from build123d import *

# Parameters (mm, degrees)
F1_DEPTH = 10
F3_D     = 10
F4_R     = 18
F5_DEPTH = 30
F7_D     = 14
F7_DEPTH = 18
F7_TIP   = 4.2060243332


with BuildPart() as f1:
    # F0 (on Top) → F1 (new body, symmetric)
    with BuildSketch(Plane.XY):
        with BuildLine():
            ThreePointArc((10.7142857143, 22.5876975726), (21.1288563682, 13.3630620956), (25, 0))
            ThreePointArc((25, 0), (29.6547751618, 8.4515425473), (39.2857142857, 9.0350790291))
            Line((39.2857142857, 9.0350790291), (10.7142857143, 22.5876975726))
        make_face()
        with BuildLine():
            ThreePointArc((39.2857142857, -9.0350790291), (29.6547751618, -8.4515425473), (25, 0))
            ThreePointArc((25, 0), (21.1288563682, -13.3630620956), (10.7142857143, -22.5876975726))
            Line((10.7142857143, -22.5876975726), (39.2857142857, -9.0350790291))
        make_face()
        with BuildLine():
            ThreePointArc((-25, 0), (-21.1288563682, 13.3630620956), (-10.7142857143, 22.5876975726))
            Line((-10.7142857143, 22.5876975726), (-39.2857142857, 9.0350790291))
            ThreePointArc((-39.2857142857, 9.0350790291), (-29.6547751618, 8.4515425473), (-25, 0))
        make_face()
        with BuildLine():
            ThreePointArc((-39.2857142857, -9.0350790291), (-29.6547751618, -8.4515425473), (-25, 0))
            ThreePointArc((-25, 0), (-29.6547751618, 8.4515425473), (-39.2857142857, 9.0350790291))
            ThreePointArc((-39.2857142857, 9.0350790291), (-45, 0), (-39.2857142857, -9.0350790291))
        make_face()
        with BuildLine():
            ThreePointArc((39.2857142857, 9.0350790291), (29.6547751618, 8.4515425473), (25, 0))
            ThreePointArc((25, 0), (29.6547751618, -8.4515425473), (39.2857142857, -9.0350790291))
            ThreePointArc((39.2857142857, -9.0350790291), (43.4515425473, -5.3452248382), (45, 0))
            ThreePointArc((45, 0), (43.4515425473, 5.3452248382), (39.2857142857, 9.0350790291))
        make_face()
        with BuildLine():
            Line((-39.2857142857, -9.0350790291), (-10.7142857143, -22.5876975726))
            ThreePointArc((-10.7142857143, -22.5876975726), (-21.1288563682, -13.3630620956), (-25, 0))
            ThreePointArc((-25, 0), (-29.6547751618, -8.4515425473), (-39.2857142857, -9.0350790291))
        make_face()
        with BuildLine():
            ThreePointArc((10.7142857143, -22.5876975726), (21.1288563682, -13.3630620956), (25, 0))
            ThreePointArc((25, 0), (21.1288563682, 13.3630620956), (10.7142857143, 22.5876975726))
            ThreePointArc((10.7142857143, 22.5876975726), (0, 25), (-10.7142857143, 22.5876975726))
            ThreePointArc((-10.7142857143, 22.5876975726), (-21.1288563682, 13.3630620956), (-25, 0))
            ThreePointArc((-25, 0), (-21.1288563682, -13.3630620956), (-10.7142857143, -22.5876975726))
            ThreePointArc((-10.7142857143, -22.5876975726), (0, -25), (10.7142857143, -22.5876975726))
        make_face()
    extrude(amount=F1_DEPTH, both=True)

    # F3 (through all)
    with Locations(Plane.XY.offset(10)):
        with Locations((-35, 0), (35, 0)):
            Hole(F3_D / 2)

    # F4 (on face) → F5 (join)
    with BuildSketch(Plane.XY.offset(10)):
        Circle(F4_R)
    extrude(amount=F5_DEPTH)

    # F7
    with Locations(Plane.XY.offset(40)):
        with Locations((0, 0)):
            Hole(F7_D / 2, depth=F7_DEPTH)
            with Locations((0, 0, -(F7_DEPTH + F7_TIP / 2))):  # 118° drill point
                Cone(0, F7_D / 2, F7_TIP, mode=Mode.SUBTRACT)


solid = f1.part
Work out the finished part from the listing and answer in its coordinate system (mm). A direction names the side the tool comes from. Give positions to 0.01 mm unless a question says otherwise; leave off trailing zeros. Loops run counter-clockwise (first coordinate to the right, second up) from the corner with the lowest first, then second, coordinate; pieces in that order, holes last. Notation, with made-up numbers: (41, 38.25) - (61, 38.25) arc R21 cw to (61, 52.25) - close; hole circle Ø9 at (1.5, 84.25). An arc over 180 degrees is marked (long way). Answer in a Markdown table with one row per item.
(1) Section C-C (y = -4) is taken. State how many separate pieces and enclosed holes the cut face has, and give its area (3 significant figures).
Results list:
| item | result |
|---|---|
| separate pieces | 3 |
| enclosed holes | 0 |
| area | 2,360 mm² |
(2) Consider L1, parallel to Y at x = 0, z = 30; L2, parallel to Z at x = -28, y = 1; L3, parallel to Y at x = -35, z = -4. Determine where each line is inside the solid, lowest interval first. Write a range as [from, to].
Results list:
| item | result |
|---|---|
| L1 | y = [-18, -7], [7, 18] |
| L2 | z = [-10, 10] |
| L3 | y = [-11.07, -5], [5, 11.07] |
(3) For a pull along Y with two mould halves and no side action, classify faces 3 (the face through (-6.466, -2.681, 30.874)), 4 (the face through (-1, 0, -10)), 5 (the face through (-24.8, 15.906, 0.14)), 6 (the face through (0, -25, 0)) as pulls with the +Y half, pulls with the -Y half, needs draft (parallel to the pull), parting line crosses it, or undercut.
Results list:
| item | result |
|---|---|
| face 3 | undercut |
| face 4 | needs draft |
| face 5 | pulls with the +Y half |
| face 6 | pulls with the -Y half |
(4) A tool of negligible diameter and unlimited length cuts with its end or side. For faces 1 (the face through (-2.343, 17.847, 24.79)), 2 (the face through (25.2, 15.717, 0.14)), from which of +Z, -Z, +X, -X, +Y, -Y can it reach the whole face along a straight path? Write none if from no direction.
Results list:
| item | result |
|---|---|
| face 1 | +Z |
| face 2 | +Z, -Z, +X, +Y |
(5) Flat-ended cylindrical pins translate along their axes: pin 1 Ø10 at (x, z) = (-15, 19.5) entering from -Y; pin 2 Ø3 at (y, z) = (0.5, 23) entering from +X; pin 3 Ø16 at (x, y) = (35, 0) entering from +Z. Find the tip coordinate at first contact, or state that the pin passes through.
Results list:
| item | result |
|---|---|
| pin 1 | stops at y = -14.97 |
| pin 2 | stops at x = 18 |
| pin 3 | stops at z = 10 |
(6) Section A-A (z = 3.5) is taken. Give the vertices of the cut face in (x, y), and give its area (3 significant figures).
Results list:
| item | result |
|---|---|
| outline | (-39.29, -9.04) - (-10.71, -22.59) arc R25 ccw to (10.71, -22.59) - (39.29, -9.04) arc R10 ccw to (39.29, 9.04) - (10.71, 22.59) arc R25 ccw to (-10.71, 22.59) - (-39.29, 9.04) arc R10 ccw to start; hole circle Ø10 at (-35, 0); hole circle Ø10 at (35, 0) |
| area | 2,840 mm² |
(7) Section B-B (x = 35) is taken. Give the vertices of the cut face in (y, z), and give its area (3 significant figures).
Results list:
| item | result |
|---|---|
| outline | (-11.07, -10) - (-5, -10) - (-5, 10) - (-11.07, 10) - close; (5, -10) - (11.07, -10) - (11.07, 10) - (5, 10) - close |
| area | 243 mm² |
(8) Section D-D (z = 28) is taken. Give the vertices of the cut face in (x, y).
Results list:
| item | result |
|---|---|
| outline | circle Ø36 at (0, 0); hole circle Ø14 at (0, 0) |
